Read the model definition and answer for the solid it produces. Units are mm, in the model's axes. Face numbers are marked on the shaded views. A direction names the side the tool comes from. Round coordinates to 2 decimals unless told otherwise and drop trailing zeros. Write each loop counter-clockwise with the first axis right and the second up, starting at its lowest first coordinate (ties: lowest second). Pieces come first, ordered by that corner, then holes.
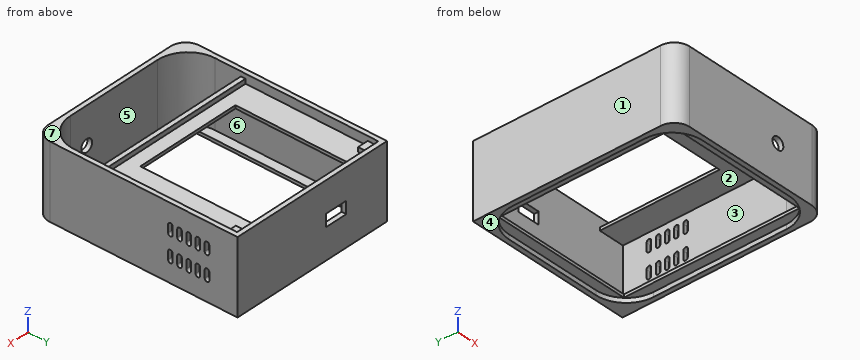
from build123d import *

# Parameters (mm, degrees)
SKETCH_1_W          = 110
SKETCH_1_H          = 133
EXTRUDE_1_DEPTH     = 48
SKETCH_2_W          = 104
SKETCH_2_H          = 127
CUT_EXTRUDE_1_DEPTH = 50
SKETCH_3_W          = 104
SKETCH_3_H          = 2
EXTRUDE_2_DEPTH     = 90
CUT_EXTRUDE_2_REACH = 97.975
SKETCH_4_W          = 70
SKETCH_4_H          = 70
SKETCH_5_W          = 104
SKETCH_5_H          = 3
EXTRUDE_3_DEPTH     = 3
SKETCH_6_W          = 15
SKETCH_6_H          = 8
CUT_EXTRUDE_3_DEPTH = 10
SKETCH_8_W          = 70
SKETCH_8_H          = 8.5
CUT_EXTRUDE_4_DEPTH = 2
EXTRUDE_4_REACH     = 136.816
SKETCH_9_W          = 2
SKETCH_9_H          = 127
SKETCH_10_W         = 92
SKETCH_10_H         = 115
CUT_EXTRUDE_5_DEPTH = 8
FILLET_10_R         = 10
FILLET_11_R         = 20
FILLET_12_R         = 20
FILLET_13_R         = 10
FILLET_14_R         = 20
FILLET_15_R         = 20
FILLET_16_R         = 20
SKETCH_11_W         = 7
SKETCH_11_H         = 7
EXTRUDE_5_DEPTH     = 3
SKETCH_12_R         = 4
CUT_EXTRUDE_6_DEPTH = 3
CUT_EXTRUDE_7_DEPTH = 3


with BuildPart() as part:
    # 草图1 → 凸台-拉伸1 (new body)
    with BuildSketch(Plane.XY):
        Rectangle(SKETCH_1_W, SKETCH_1_H)
    extrude(amount=EXTRUDE_1_DEPTH)

    # 草图2 → 切除-拉伸1 (cut)
    with BuildSketch(Plane.XY.offset(48)):
        Rectangle(SKETCH_2_W, SKETCH_2_H)
    extrude(amount=-CUT_EXTRUDE_1_DEPTH, mode=Mode.SUBTRACT)

    # 草图3 → 凸台-拉伸2 (add)
    with BuildSketch(Plane.XZ.offset(-63.5)):
        with Locations((0, 41)):
            Rectangle(SKETCH_3_W, SKETCH_3_H)
    extrude(amount=EXTRUDE_2_DEPTH)

    # 草图4 → 切除-拉伸2 (cut, up to next)
    with BuildSketch(Plane.XY.offset(42), mode=Mode.PRIVATE) as cut_extrude_2_sk1:
        with Locations((0, 20)):
            Rectangle(SKETCH_4_W, SKETCH_4_H)
    cut_extrude_2_tool1 = extrude(cut_extrude_2_sk1.sketch, amount=-CUT_EXTRUDE_2_REACH, mode=Mode.PRIVATE) & part.part
    add(cut_extrude_2_tool1.solids().sort_by_distance((0, 20, 42))[0], mode=Mode.SUBTRACT)

    # 草图5 → 凸台-拉伸3 (add)
    with BuildSketch(Plane.XY.offset(42)):
        with Locations((0, -25)):
            Rectangle(SKETCH_5_W, SKETCH_5_H)
    extrude(amount=EXTRUDE_3_DEPTH)

    # 草图6 → 切除-拉伸3 (cut)
    with BuildSketch(Plane(origin=(0, 66.5, 0), x_dir=(1, 0, 0), z_dir=(0, 1, 0))):
        with Locations((-17.5, -24)):
            Rectangle(SKETCH_6_W, SKETCH_6_H)
    extrude(amount=-CUT_EXTRUDE_3_DEPTH, mode=Mode.SUBTRACT)

    # 草图8 → 切除-拉伸4 (cut)
    with BuildSketch(Plane.XY.offset(42)):
        with Locations((0, 59.25)):
            Rectangle(SKETCH_8_W, SKETCH_8_H)
    extrude(amount=-CUT_EXTRUDE_4_DEPTH, mode=Mode.SUBTRACT)

    # 草图9 → 凸台-拉伸4 (add, up to next)
    with BuildSketch(Plane.ZY.offset(-52), mode=Mode.PRIVATE) as extrude_4_sk1:
        with Locations((4, 0)):
            Rectangle(SKETCH_9_W, SKETCH_9_H)
    extrude_4_tool1 = extrude(extrude_4_sk1.sketch, amount=EXTRUDE_4_REACH, mode=Mode.PRIVATE) - part.part
    add(extrude_4_tool1.solids().sort_by_distance((52, 0, 4))[0])

    # 草图10 → 切除-拉伸5 (cut)
    with BuildSketch(Plane(origin=(0, 0, 3), x_dir=(-1, 0, 0), z_dir=(0, 0, -1))):
        Rectangle(SKETCH_10_W, SKETCH_10_H)
    extrude(amount=-CUT_EXTRUDE_5_DEPTH, mode=Mode.SUBTRACT)

    # 圆角10
    fillet_10_edges = [part.edges().sort_by_distance(p)[0] for p in [
        (-55, -66.5, 24),
    ]]
    fillet(fillet_10_edges, radius=FILLET_10_R)

    # 圆角11
    fillet_11_edges = [part.edges().sort_by_distance(p)[0] for p in [
        (-52, -63.5, 1.5),
    ]]
    fillet(fillet_11_edges, radius=FILLET_11_R)

    # 圆角12
    fillet_12_edges = [part.edges().sort_by_distance(p)[0] for p in [
        (52, -63.5, 1.5),
    ]]
    fillet(fillet_12_edges, radius=FILLET_12_R)

    # 圆角13
    fillet_13_edges = [part.edges().sort_by_distance(p)[0] for p in [
        (55, -66.5, 24),
    ]]
    fillet(fillet_13_edges, radius=FILLET_13_R)

    # 圆角14
    fillet_14_edges = [part.edges().sort_by_distance(p)[0] for p in [
        (-52, 63.5, 1.5),
        (52, 63.5, 1.5),
    ]]
    fillet(fillet_14_edges, radius=FILLET_14_R)

    # 圆角15
    fillet_15_edges = [part.edges().sort_by_distance(p)[0] for p in [
        (52, -63.5, 26.5),
    ]]
    fillet(fillet_15_edges, radius=FILLET_15_R)

    # 圆角16
    fillet_16_edges = [part.edges().sort_by_distance(p)[0] for p in [
        (-52, -63.5, 26.5),
    ]]
    fillet(fillet_16_edges, radius=FILLET_16_R)

    # 草图11 → 凸台-拉伸5 (add)
    with BuildSketch(Plane.XY.offset(42)):
        with Locations((48.5, 60)):
            Rectangle(SKETCH_11_W, SKETCH_11_H)
        with Locations((-48.5, 60)):
            Rectangle(SKETCH_11_W, SKETCH_11_H)
    extrude(amount=EXTRUDE_5_DEPTH)

    # 草图12 → 切除-拉伸6 (cut)
    with BuildSketch(Plane.XZ.offset(66.5)):
        with Locations(Location((20, 24, 0), (0, 0, 270))):
            Circle(SKETCH_12_R)
    extrude(amount=-CUT_EXTRUDE_6_DEPTH, mode=Mode.SUBTRACT)

    # 草图13 → 切除-拉伸7 (cut)
    with BuildSketch(Plane.ZY.offset(-52)):
        with BuildLine():
            Line((13.5, 48), (18.5, 48))
            ThreePointArc((18.5, 48), (20, 46.5), (18.5, 45))
            Line((18.5, 45), (13.5, 45))
            ThreePointArc((13.5, 45), (12, 46.5), (13.5, 48))
        make_face()
        with BuildLine():
            Line((34.5, 48), (29.5, 48))
            ThreePointArc((29.5, 48), (28, 46.5), (29.5, 45))
            Line((29.5, 45), (34.5, 45))
            ThreePointArc((34.5, 45), (36, 46.5), (34.5, 48))
        make_face()
        with BuildLine():
            Line((13.5, 42), (18.5, 42))
            ThreePointArc((18.5, 42), (20, 40.5), (18.5, 39))
            Line((18.5, 39), (13.5, 39))
            ThreePointArc((13.5, 39), (12, 40.5), (13.5, 42))
        make_face()
        with BuildLine():
            Line((13.5, 36), (18.5, 36))
            ThreePointArc((18.5, 36), (20, 34.5), (18.5, 33))
            Line((18.5, 33), (13.5, 33))
            ThreePointArc((13.5, 33), (12, 34.5), (13.5, 36))
        make_face()
        with BuildLine():
            Line((13.5, 30), (18.5, 30))
            ThreePointArc((18.5, 30), (20, 28.5), (18.5, 27))
            Line((18.5, 27), (13.5, 27))
            ThreePointArc((13.5, 27), (12, 28.5), (13.5, 30))
        make_face()
        with BuildLine():
            Line((13.5, 24), (18.5, 24))
            ThreePointArc((18.5, 24), (20, 22.5), (18.5, 21))
            Line((18.5, 21), (13.5, 21))
            ThreePointArc((13.5, 21), (12, 22.5), (13.5, 24))
        make_face()
        with BuildLine():
            Line((34.5, 24), (29.5, 24))
            ThreePointArc((29.5, 24), (28, 22.5), (29.5, 21))
            Line((29.5, 21), (34.5, 21))
            ThreePointArc((34.5, 21), (36, 22.5), (34.5, 24))
        make_face()
        with BuildLine():
            Line((34.5, 30), (29.5, 30))
            ThreePointArc((29.5, 30), (28, 28.5), (29.5, 27))
            Line((29.5, 27), (34.5, 27))
            ThreePointArc((34.5, 27), (36, 28.5), (34.5, 30))
        make_face()
        with BuildLine():
            Line((34.5, 36), (29.5, 36))
            ThreePointArc((29.5, 36), (28, 34.5), (29.5, 33))
            Line((29.5, 33), (34.5, 33))
            ThreePointArc((34.5, 33), (36, 34.5), (34.5, 36))
        make_face()
        with BuildLine():
            Line((34.5, 42), (29.5, 42))
            ThreePointArc((29.5, 42), (28, 40.5), (29.5, 39))
            Line((29.5, 39), (34.5, 39))
            ThreePointArc((34.5, 39), (36, 40.5), (34.5, 42))
        make_face()
    extrude(amount=-CUT_EXTRUDE_7_DEPTH, mode=Mode.SUBTRACT)


solid = part.part
Q1. Section A-A (x = 20) is taken. Determine the outline of the cut face in (y, z).
Verdict:
outline: (-66.5, 0) - (-63.5, 0) - (-63.5, 3) - (-57.5, 3) - (-57.5, 5) - (-63.5, 5) - (-63.5, 20) - (-66.5, 20) - close; (-66.5, 28) - (-63.5, 28) - (-63.5, 48) - (-66.5, 48) - close; (-26.5, 40) - (-15, 40) - (-15, 42) - (-23.5, 42) - (-23.5, 45) - (-26.5, 45) - close; (57.5, 3) - (63.5, 3) - (63.5, 0) - (66.5, 0) - (66.5, 48) - (63.5, 48) - (63.5, 5) - (57.5, 5) - close
Q2. Flat-ended cylindrical pins translate along their axes: pin 1 Ø0.9 at (x, z) = (53, 31) entering from -Y; pin 2 Ø2 at (x, y) = (48.5, 59) entering from +Z; pin 3 Ø10 at (x, y) = (-6, -18) entering from -Z. Find the tip coordinate at first contact, or state that the pin passes through.
Verdict:
pin 1: stops at y = -63.06
pin 2: stops at z = 45
pin 3: stops at z = 40
Q3. Section C-C (z = 24) is taken. Determine the outline of the cut face in (x, y).
Verdict:
outline: (-55, -56.5) arc R10 ccw to (-45, -66.5) - (16, -66.5) - (16, -63.5) - (-32, -63.5) arc R20 cw to (-52, -43.5) - (-52, 63.5) - (-25, 63.5) - (-25, 66.5) - (-55, 66.5) - close; (-10, 63.5) - (52, 63.5) - (52, -43.5) arc R20 cw to (32, -63.5) - (24, -63.5) - (24, -66.5) - (45, -66.5) arc R10 ccw to (55, -56.5) - (55, 66.5) - (-10, 66.5) - close
Q4. Straight lines are drawn through the part: probe 1 along Y at (x, z) = (30, 9); probe 2 along X at (y, z) = (52, 10.5); probe 3 along Y at (x, z) = (-44, 42.5). For each, find the intervals that lie inside material, in ascending order.
Verdict:
probe 1: y = -66.5 to -63.5, 63.5 to 66.5
probe 2: x = -55 to -52, 52 to 55
probe 3: y = -66.5 to -59.5, -26.5 to -23.5, 63.5 to 66.5
Q5. Which of the six approach directions +Z, -Z, +X, -X, +Y, -Y give full straight-line access (tool end or side, diameter ignored) to the marked faces 5, 6 and 7?
Verdict:
face 5: +Z
face 6: none
face 7: +Z, +X, -X, +Y, -Y
Q6. Section D-D (y = -41) is taken. Determine the outline of the cut face in (x, z).
Verdict:
outline: (-55, 0) - (-52, 0) - (-52, 3) - (-46, 3) - (-46, 5) - (-52, 5) - (-52, 48) - (-55, 48) - close; (46, 3) - (52, 3) - (52, 0) - (55, 0) - (55, 48) - (52, 48) - (52, 5) - (46, 5) - close
Q7. Section B-B (z = 9) is taken. Determine the outline of the cut face in (x, y).
Verdict:
outline: (-55, -56.5) arc R10 ccw to (-45, -66.5) - (45, -66.5) arc R10 ccw to (55, -56.5) - (55, 66.5) - (-55, 66.5) - close; hole (-52, -43.5) arc R20 ccw to (-32, -63.5) - (32, -63.5) arc R20 ccw to (52, -43.5) - (52, 63.5) - (-52, 63.5) - close
Q8. Determine the mould class of the marked faces 1, 2, 3 and 4 for opening direction Z: pulls with the +Z half, pulls with the -Z half, needs draft (parallel to the pull), parting line crosses it, or undercut.
Verdict:
face 1: needs draft
face 2: undercut
face 3: undercut
face 4: pulls with the -Z half
